Study the drawing (mm; zero at the part's minimum x, y, z) and answer. Coordinates: 2 decimals unless noted, no trailing zeros. Order: outer loops, then holes, each group sorted by start corner. A loop starts at its lowest first (then second) coordinate and runs counter-clockwise, first axis right, second up. Notation, with made-up numbers: (34.25, 3) -> (92.25, 3) arc R36 ccw to (92.25, 42) -> close; hole circle Ø1 at (-17.75, -12). An arc over 180 degrees is marked (long way). Write each question's results on one line, items separated by ' | '. Start each with the question number.
(1) The part is cut by section B-B, the plane y = 11. Give the vertices of the cut face in (x, z).
(2) The part is cut by section C-C, the plane x = 37. Give the vertices of the cut face in (y, z), then the cut area to 3 significant figures.
(3) The part is cut by section D-D, the plane x = 27. Count the separate pieces of the cut face and the enclosed holes in it, then the cut area to 3 significant figures.
(4) Determine the mould class of the marked faces 1, 2 and 3 for opening direction Z: +Z half, -Z half, draft (parallel to the pull), parting line (faces both ways), or undercut.
(5) Straight lines are drawn through the part: L1, parallel to Z at x = 3.5, y = 3; L2, parallel to X at y = 1.7, z = 34 (3 decimals). For each, find the intervals that lie inside material, in ascending order.
(6) Given pin 1 (15 mm diameter, centred on x = 29, z = 29, fed in from +Y); pin 2 (3 mm diameter, centred on x = 27, z = 20, fed in from -Y), each flat-ended and moving along its own axis, determine where each tip first touches the part or whether it passes through.
(7) The part is cut by section A-A, the plane z = 3.5. Give the vertices of the cut face in (x, y).
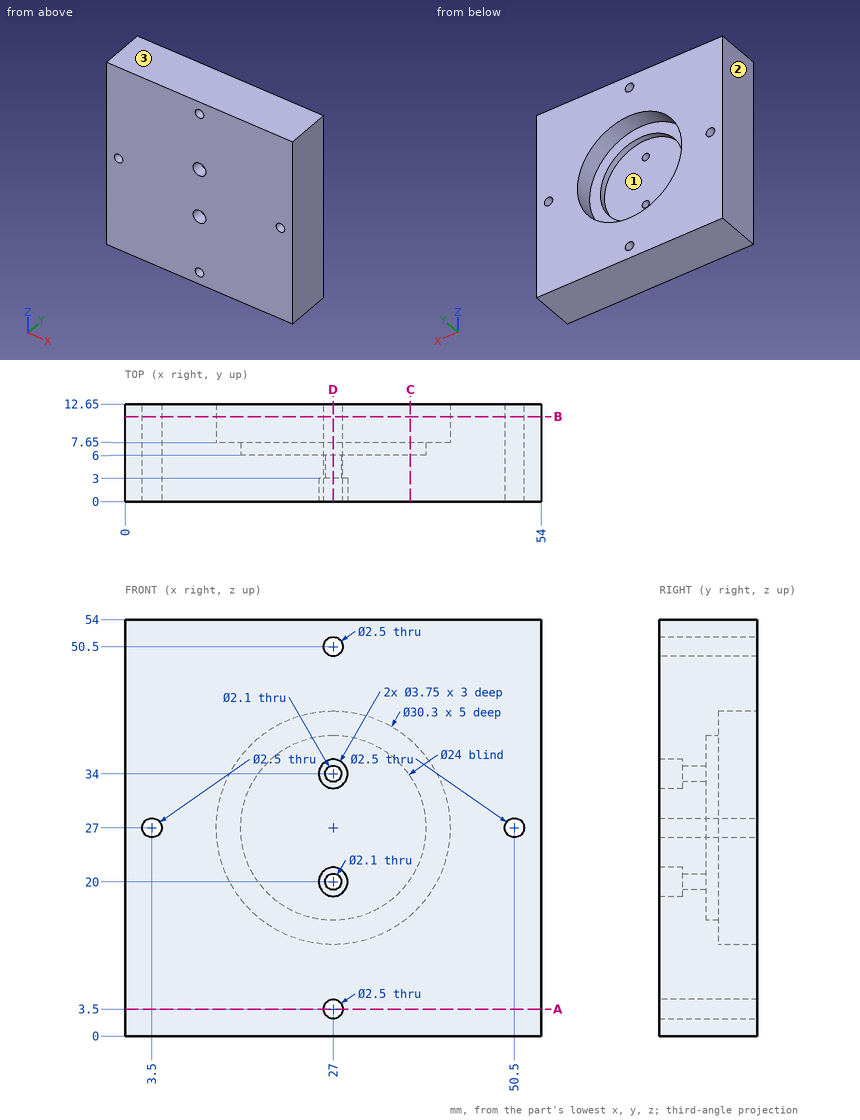
Established:
1) outline: (0, 0) -> (54, 0) -> (54, 54) -> (0, 54) -> close; hole circle Ø2.5 at (3.5, 27); hole circle Ø30.3 at (27, 27); hole circle Ø2.5 at (27, 3.5); hole circle Ø2.5 at (27, 50.5); hole circle Ø2.5 at (50.5, 27)
2) outline: (0, 0) -> (12.65, 0) -> (12.65, 15.62) -> (7.65, 15.62) -> (7.65, 20.37) -> (6, 20.37) -> (6, 33.63) -> (7.65, 33.63) -> (7.65, 38.38) -> (12.65, 38.38) -> (12.65, 54) -> (0, 54) -> close | area: 547 mm^2
3) separate pieces: 5 | enclosed holes: 0 | area: 394 mm^2
4) face 1: undercut | face 2: draft | face 3: +Z half
5) L1: z = 0 to 25.75, 28.25 to 54 | L2: x = 0 to 25.125, 28.875 to 54
6) pin 1: stops at y = 6 | pin 2: stops at y = 3
7) outline: (0, 0) -> (25.75, 0) -> (25.75, 12.65) -> (0, 12.65) -> close; (28.25, 0) -> (54, 0) -> (54, 12.65) -> (28.25, 12.65) -> close
